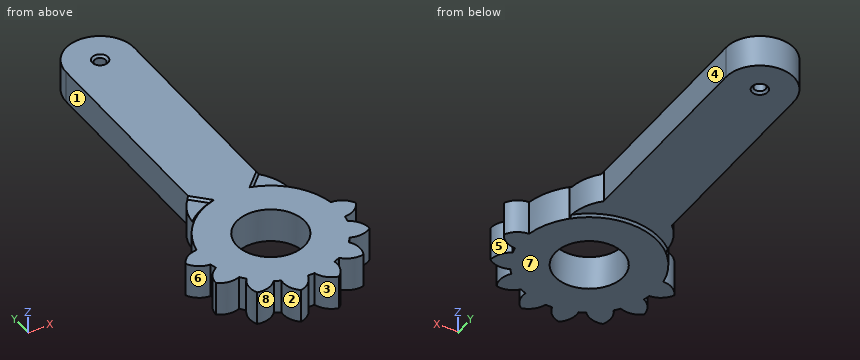
```python
from build123d import *

# Parameters (mm, degrees)
SKETCH2_R           = 30
SKETCH2_R_2         = 15
BOSS_EXTRUDE1_DEPTH = 7.5
BOSS_EXTRUDE2_DEPTH = 6.5
CHAMFER2_SIZE       = 1
BOSS_EXTRUDE3_DEPTH = 14
CHAMFER3_SIZE       = 1
SKETCH6_R           = 2.5
CUT_EXTRUDE1_DEPTH  = 14
CHAMFER4_SIZE       = 1
CHAMFER5_SIZE       = 1
BOSS_EXTRUDE4_DEPTH = 15


# Some blends are built 0.0001 mm under size
with BuildPart() as part:
    # Sketch2 → Boss-Extrude1 (new, symmetric)
    with BuildSketch(Plane.XY):
        Circle(SKETCH2_R)
        Circle(SKETCH2_R_2, mode=Mode.SUBTRACT)
    extrude(amount=BOSS_EXTRUDE1_DEPTH, both=True)

    # Sketch4 → Boss-Extrude2 (add, symmetric)
    with BuildSketch(Plane.XY):
        with BuildLine():
            ThreePointArc((-21.213203436, 21.213203436), (0, 42.343834222), (21.213203436, 21.213203436))
            ThreePointArc((21.213203436, 21.213203436), (0, 30), (-21.213203436, 21.213203436))
        make_face()
    extrude(amount=BOSS_EXTRUDE2_DEPTH, both=True)

    # Chamfer2
    chamfer2_edges = [part.edges().sort_by_distance(p)[0] for p in [
        (0, 30, -6.5),
        (0, 30, 6.5),
    ]]
    chamfer(chamfer2_edges, length=CHAMFER2_SIZE - 0.0001)  # a hair under: the kernel refuses the full size

    # Sketch5 → Boss-Extrude3 (add)
    with BuildSketch(Plane(origin=(0, 0, -6.5), x_dir=(-1, 0, 0), z_dir=(0, 0, -1))):
        with BuildLine():
            Line((0, 21.130469451), (-15.000114081, 36.130583532))
            Line((-15.000114081, 36.130583532), (-15.000114081, 126.716493473))
            ThreePointArc((-15.000114081, 126.716493473), (0, 141.716607555), (15.000114081, 126.716493473))
            Line((15.000114081, 126.716493473), (15.000114081, 36.130583532))
            Line((15.000114081, 36.130583532), (0, 21.130469451))
        make_face()
    extrude(amount=-BOSS_EXTRUDE3_DEPTH)

    # Chamfer3
    # the kernel refuses this chamfer: 1 mm, written as the material it adds along each edge
    with BuildSketch(Plane(origin=(6.82237013, 27.952839581, 6.5), x_dir=(0.7068394360706772, -0.7068394360706699, -0.02749587661058651), z_dir=(0.7071067811865439, 0.7071067811865512, 0))) as chamfer3_piece_1_section:
        Polygon((CHAMFER3_SIZE * 0.999621916911, -CHAMFER3_SIZE * 0.0274958766106), (-CHAMFER3_SIZE * 0.0274958766106, -CHAMFER3_SIZE * 0.999621916911), (0, 0), align=None)
    chamfer3_piece_1 = extrude(amount=14.136759393, mode=Mode.PRIVATE)
    chamfer3_piece_1 = chamfer3_piece_1 & Plane(origin=(0, 21.130469451, 6.845303942), x_dir=(-0.9999923946286841, 0.003900087792649399, 0), z_dir=(0, 0, 1)) * Cylinder(21.213364771, 33, mode=Mode.PRIVATE)
    add(chamfer3_piece_1)
    with BuildSketch(Plane(origin=(-16.818568561, 37.949038012, 6.5), x_dir=(0.019442520806013823, 0.019442520806013757, 0.9996219169112968), z_dir=(0.7071067811865464, -0.7071067811865487, 0))) as chamfer3_piece_2_section:
        Polygon((CHAMFER3_SIZE * 0.999621916911, CHAMFER3_SIZE * 0.0274958766106), (-CHAMFER3_SIZE * 0.0274958766106, CHAMFER3_SIZE * 0.999621916911), (0, 0), align=None)
    chamfer3_piece_2 = extrude(amount=14.136759393, mode=Mode.PRIVATE)
    chamfer3_piece_2 = chamfer3_piece_2 & Plane(origin=(0, 21.130469451, 6.750596564), x_dir=(-0.9999923946286841, 0.003900087792649399, 0), z_dir=(0, 0, 1)) * Cylinder(21.213364771, 33, mode=Mode.PRIVATE)
    add(chamfer3_piece_2)

    # Sketch6 → Cut-Extrude1 (cut)
    with BuildSketch(Plane.XY.offset(7.5)):
        with Locations((0, 126.716493473)):
            Circle(SKETCH6_R)
    extrude(amount=-CUT_EXTRUDE1_DEPTH, mode=Mode.SUBTRACT)

    # Chamfer4
    chamfer4_edges = [part.edges().sort_by_distance(p)[0] for p in [
        (-2.5, 126.716493473, 7.5),
    ]]
    chamfer(chamfer4_edges, length=CHAMFER4_SIZE)

    # Chamfer5
    chamfer5_edges = [part.edges().sort_by_distance(p)[0] for p in [
        (-2.5, 126.716493473, -6.5),
    ]]
    chamfer(chamfer5_edges, length=CHAMFER5_SIZE)

    # Sketch7 → Boss-Extrude4 (add)
    with BuildSketch(Plane.XY.offset(7.5)):
        with BuildLine():
            ThreePointArc((-29.538927614, 5.23944228), (-34.249735627, 3.72933291), (-37.5, 0))
            ThreePointArc((-37.5, 0), (-34.249735627, -3.72933291), (-29.538927614, -5.23944228))
            ThreePointArc((-29.538927614, -5.23944228), (-30, 0), (-29.538927614, 5.23944228))
        make_face()
        with BuildLine():
            ThreePointArc((-28.886962979, -8.095885983), (-32.476042442, -11.500390508), (-33.786332546, -16.270640217))
            ThreePointArc((-33.786332546, -16.270640217), (-29.239848627, -18.220416208), (-24.340345364, -17.537034743))
            ThreePointArc((-24.340345364, -17.537034743), (-27.029066037, -13.016512174), (-28.886962979, -8.095885983))
        make_face()
        with BuildLine():
            ThreePointArc((-22.513581051, -19.827724738), (-24.270070758, -24.452320542), (-23.38086757, -29.318680593))
            ThreePointArc((-23.38086757, -29.318680593), (-18.438651002, -29.102722617), (-14.3208592, -26.361202396))
            ThreePointArc((-14.3208592, -26.361202396), (-18.704694056, -23.454944474), (-22.513581051, -19.827724738))
        make_face()
        with BuildLine():
            ThreePointArc((-11.681108284, -27.632439437), (-11.257113908, -32.561168606), (-8.344535023, -36.559796707))
            ThreePointArc((-8.344535023, -36.559796707), (-3.985452411, -34.22087789), (-1.464951237, -29.964210617))
            ThreePointArc((-1.464951237, -29.964210617), (-6.675628019, -29.247837365), (-11.681108284, -27.632439437))
        make_face()
        with BuildLine():
            ThreePointArc((1.464951237, -29.964210617), (3.985452411, -34.22087789), (8.344535023, -36.559796707))
            ThreePointArc((8.344535023, -36.559796707), (11.257113908, -32.561168606), (11.681108284, -27.632439437))
            ThreePointArc((11.681108284, -27.632439437), (6.675628019, -29.247837365), (1.464951237, -29.964210617))
        make_face()
        with BuildLine():
            ThreePointArc((14.3208592, -26.361202396), (18.438651002, -29.102722617), (23.38086757, -29.318680593))
            ThreePointArc((23.38086757, -29.318680593), (24.270070758, -24.452320542), (22.513581051, -19.827724738))
            ThreePointArc((22.513581051, -19.827724738), (18.704694056, -23.454944474), (14.3208592, -26.361202396))
        make_face()
        with BuildLine():
            ThreePointArc((33.786332546, -16.270640217), (32.476042442, -11.500390508), (28.886962979, -8.095885983))
            ThreePointArc((28.886962979, -8.095885983), (27.029066037, -13.016512174), (24.340345364, -17.537034743))
            ThreePointArc((24.340345364, -17.537034743), (29.239848627, -18.220416208), (33.786332546, -16.270640217))
        make_face()
        with BuildLine():
            ThreePointArc((29.538927614, 5.23944228), (29.884509603, 2.629845202), (30, 0))
            ThreePointArc((30, 0), (29.884509603, -2.629845202), (29.538927614, -5.23944228))
            ThreePointArc((29.538927614, -5.23944228), (34.249735627, -3.72933291), (37.5, 0))
            ThreePointArc((37.5, 0), (34.249735627, 3.72933291), (29.538927614, 5.23944228))
        make_face()
    extrude(amount=-BOSS_EXTRUDE4_DEPTH)


solid = part.part
```
Geometry check sheet. Reference: the model listing, model coordinates, mm. Face numbers are marked on the shaded views. A direction names the side the tool comes from. Round coordinates to 2 decimals unless told otherwise and drop trailing zeros. Loops run counter-clockwise (first coordinate to the right, second up) from the corner with the lowest first, then second, coordinate; pieces in that order, holes last. Notation, with made-up numbers: M 84.25,70.25 L 89.25,70.25 A6 cw 89.25,77.25 Z; hole C -3,88 d7. An arc over 180 degrees is marked long. Return JSON: item names as keys, results as strings. Group by question number.
(1) Go/stop test with flat-tipped pins: pin 1 (21 mm diameter, centred on x = 7, y = 80, fed in from -Z); pin 2 (6 mm diameter, centred on x = 4, z = 3.5, fed in from +Y); pin 3 (2 mm diameter, centred on x = -13, z = 0.5, fed in from +Y); pin 4 (3 mm diameter, centred on x = 0, y = 126.72, fed in from -Z). Record where each tip stops, or that it passes through.
(2) Set-up check for the marked faces 1, 2, 3, 4 and 5: record each of +Z, -Z, +X, -X, +Y, -Y from which the full face is reachable in a straight line by a thin tool's end or side.
(3) Section check D-D, the plane y = -21.5. Enter the section's corners in (x, z), and give its area (3 significant figures).
(4) Scan lines: line 1 along Y through (x, z) = (0, -1); line 2 along X through (y, z) = (-27, -1.75); line 3 along X through (y, z) = (111, 0.75). Record each from-to range of solid material in increasing order. Write a range as [from, to].
(5) Mould release check, pull along X, two halves, no side actions. Record for the marked faces 6, 7 and 8: pulls with the +X half, pulls with the -X half, needs draft (parallel to the pull), parting line crosses it, or undercut.
(6) Section check B-B, the plane y = 2. Enter the section's corners in (x, z), and give its area (3 significant figures).
(7) Section check C-C, the plane y = 51. Enter the section's corners in (x, z), and give its area (3 significant figures).
(8) Section check A-A, the plane z = 0. Give the number of separate pieces and of enclosed holes in the cut face, and give its area (3 significant figures).
Data:
{
 "1": {"pin 1": "z = -6.5", "pin 2": "y = 141.68", "pin 3": "y = 135.72", "pin 4": "through"},
 "2": {"face 1": "+Z, -Z, -X, +Y", "face 2": "+Z, -Z", "face 3": "+Z, -Z, -Y", "face 4": "+Z, -Z, +X, +Y", "face 5": "+Z, -Z, +X"},
 "3": {"outline": "M -23.49,-7.5 L 23.49,-7.5 L 23.49,7.5 L -23.49,7.5 Z", "area": "705 mm²"},
 "4": {"line 1": "[-30, -15], [15, 124.22], [129.22, 141.72]", "line 2": "[-24.15, -14.93], [-13.08, 13.08], [14.93, 24.15]", "line 3": "[-15, 15]"},
 "5": {"face 6": "pulls with the -X half", "face 7": "needs draft", "face 8": "undercut"},
 "6": {"outline": "M -36.2,-7.5 L -14.87,-7.5 L -14.87,7.5 L -36.2,7.5 Z; M 14.87,-7.5 L 36.2,-7.5 L 36.2,7.5 L 14.87,7.5 Z", "area": "640 mm²"},
 "7": {"outline": "M -15,-6.5 L 15,-6.5 L 15,7.5 L -15,7.5 Z", "area": "420 mm²"},
 "8": {"separate pieces": "1", "enclosed holes": "2", "area": "5,940 mm²"}
}
